Work out the finished part from the listing and answer in its coordinate system (mm). Face numbers are marked on the shaded views. A direction names the side the tool comes from. Coordinates: 2 decimals unless noted, no trailing zeros. Order: outer loops, then holes, each group sorted by start corner. A loop starts at its lowest first (then second) coordinate and runs counter-clockwise, first axis right, second up.
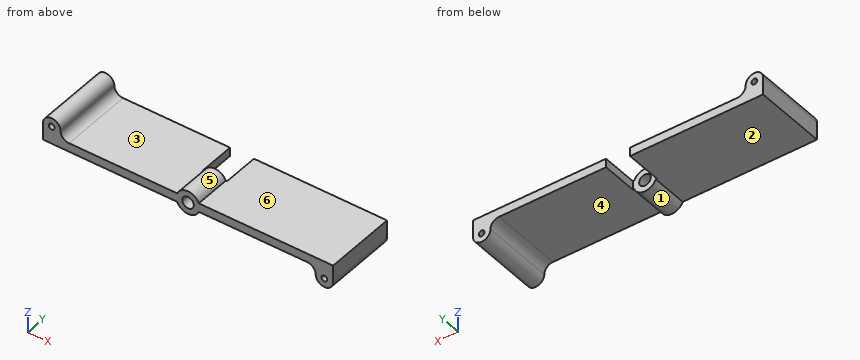
```python
from build123d import *

# Parameters (mm, degrees)
F0_R     = 1
F0_R_2   = 2
F1_DEPTH = 25
F2_W     = 8.25
F2_H     = 12.5
F3_DEPTH = 12.5


with BuildPart() as f1:
    # F0 (on Front) → F1 (new body)
    with BuildSketch(Plane.XZ):
        with BuildLine():
            Line((-3.708099, 1.5), (-41, 1.5))
            ThreePointArc((-41, 1.5), (-43.12132, 2.37868), (-44, 4.5))
            ThreePointArc((-44, 4.5), (-47, 7.5), (-50, 4.5))
            Line((-50, 4.5), (-50, 2.5))
            Line((-50, 2.5), (-50, 1.5))
            Line((-50, 1.5), (-50, -1.5))
            Line((-50, -1.5), (-3.708099, -1.5))
            ThreePointArc((-3.708099, -1.5), (0, -4), (3.708099, -1.5))
            Line((3.708099, -1.5), (41, -1.5))
            ThreePointArc((41, -1.5), (43.12132, -2.37868), (44, -4.5))
            ThreePointArc((44, -4.5), (47, -7.5), (50, -4.5))
            Line((50, -4.5), (50, -1.5))
            Line((50, -1.5), (50, 1.5))
            Line((50, 1.5), (3.708099, 1.5))
            ThreePointArc((3.708099, 1.5), (0, 4), (-3.708099, 1.5))
        make_face()
        with Locations((47, -4.5)):
            Circle(F0_R, mode=Mode.SUBTRACT)
        with Locations((-47, 4.5)):
            Circle(F0_R, mode=Mode.SUBTRACT)
        Circle(F0_R_2, mode=Mode.SUBTRACT)
    extrude(amount=F1_DEPTH)

    # F2 (on Top) → F3 (cut, symmetric)
    with BuildSketch(Plane.XY):
        with Locations((0, -6.25)):
            Rectangle(F2_W, F2_H)
    extrude(amount=F3_DEPTH, both=True, mode=Mode.SUBTRACT)


solid = f1.part
```
1. The part is cut by section D-D (y = -21). Determine the outline of the cut face in (x, z), plus the area to 3 significant figures.
2. The mould has two halves that part along X. Classify the marked faces 4, 5 and 6: released by +X, released by -X, zero draft, split by the parting line, or undercut.
3. The part is cut by section B-B (x = 0). Determine the outline of the cut face in (y, z).
4. For the marked faces 1, 2 and 3, determine the directions among +Z, -Z, +X, -X, +Y, -Y from which every point of the face is accessible in a straight line to the end or side of a thin tool.
5. The part is cut by section C-C (z = 0). Determine the outline of the cut face in (x, y) (3 decimals).
6. Flat-ended cylindrical pins translate along their axes: pin 1 (6 mm diameter, centred on x = -12.5, y = -12.5, fed in from +Z); pin 2 (7.5 mm diameter, centred on x = 24.5, y = -18, fed in from -Z); pin 3 (1.6 mm diameter, centred on x = -47, z = 4.5, fed in from -Y); pin 4 (4 mm diameter, centred on x = -2, z = 0, fed in from +Y). Find the tip coordinate at first contact, or state that the pin passes through.
7. Consider probe 1 along Z at (x, y) = (-47, -11); probe 2 along Z at (x, y) = (47, -5.5); probe 3 along Z at (x, y) = (13, -12.5). Determine where each line is inside the solid, lowest interval first.
8. The part is cut by section A-A (y = -2.25). Determine the outline of the cut face in (x, z) (3 decimals), plus the area to 3 significant figures.
Worked out:
1. outline: (-50, -1.5) - (-3.71, -1.5) arc R4 ccw to (3.71, -1.5) - (41, -1.5) arc R3 cw to (44, -4.5) arc R3 ccw to (50, -4.5) - (50, 1.5) - (3.71, 1.5) arc R4 ccw to (-3.71, 1.5) - (-41, 1.5) arc R3 cw to (-44, 4.5) arc R3 ccw to (-50, 4.5) - close; hole circle Ø2 at (-47, 4.5); hole circle Ø4 at (0, 0); hole circle Ø2 at (47, -4.5)
1. area: 376 mm2
2. face 4: undercut
2. face 5: undercut
2. face 6: zero draft
3. outline: (-25, -4) - (-12.5, -4) - (-12.5, -2) - (-25, -2) - close; (-25, 2) - (-12.5, 2) - (-12.5, 4) - (-25, 4) - close
4. face 1: -Z, +Y, -Y
4. face 2: -Z, -X, +Y, -Y
4. face 3: +Z, +Y, -Y
5. outline: (-50, -25) - (-2, -25) - (-2, -12.5) - (-4.125, -12.5) - (-4.125, 0) - (-50, 0) - close; (2, -25) - (50, -25) - (50, 0) - (4.125, 0) - (4.125, -12.5) - (2, -12.5) - close
6. pin 1: stops at z = 1.5
6. pin 2: stops at z = -1.5
6. pin 3: passes through
6. pin 4: stops at y = -12.5
7. probe 1: z = -1.5 to 3.5, 5.5 to 7.5
7. probe 2: z = -7.5 to -5.5, -3.5 to 1.5
7. probe 3: z = -1.5 to 1.5
8. outline: (-50, -1.5) - (-4.125, -1.5) - (-4.125, 1.5) - (-41, 1.5) arc R3 cw to (-44, 4.5) arc R3 ccw to (-50, 4.5) - close; (4.125, -1.5) - (41, -1.5) arc R3 cw to (44, -4.5) arc R3 ccw to (50, -4.5) - (50, 1.5) - (4.125, 1.5) - close; hole circle Ø2 at (-47, 4.5); hole circle Ø2 at (47, -4.5)
8. area: 337 mm2
